Read the model definition and answer for the solid it produces. Units are mm, in the model's axes. Face numbers are marked on the shaded views. A direction names the side the tool comes from. Coordinates: 2 decimals unless noted, no trailing zeros. Write each loop counter-clockwise with the first axis right and the second up, starting at its lowest first coordinate (ties: lowest second). Pieces come first, ordered by that corner, then holes. Notation, with made-up numbers: (81, 70.5) - (127, 70.5) arc R9 ccw to (127, 78.5) - close; hole circle Ø11 at (44.25, -31.75). An arc over 180 degrees is marked (long way). Return JSON: item names as keys, results as strings.
```python
from build123d import *

# Parameters (mm, degrees)
F0_R            = 7.874
F0_R_2          = 6.985
F0_R_3          = 1.397
F1_DEPTH        = 1.27
F2_DEPTH        = 28.575
F4_DEPTH        = 25.4
F4_COPIES_COUNT = 40
F5_SIZE         = 0.254


# Not quite as in the source:
# - a pattern or mirror of a feature is missing from the dataset's text; its kind, count and spacing are read off the source's solid


with BuildPart() as f1:
    # F0 (on Front) → F1 (new body, symmetric)
    with BuildSketch(Plane.XZ):
        Circle(F0_R)
        Circle(F0_R_2, mode=Mode.SUBTRACT)
        Circle(F0_R_2)
        Circle(F0_R_3, mode=Mode.SUBTRACT)
    extrude(amount=F1_DEPTH, both=True)

    # F0 (on Front) → F2 (join, symmetric)
    with BuildSketch(Plane.XZ):
        Circle(F0_R_3)
    extrude(amount=F2_DEPTH, both=True)

    # F3 (on face) → F4 (cut)
    with BuildSketch(Plane.XZ.offset(1.27)):
        with BuildLine():
            ThreePointArc((0.444322899, 7.861453629), (0, 7.874), (-0.444322899, 7.861453629))
            ThreePointArc((-0.444322899, 7.861453629), (0, 7.4295), (0.444322899, 7.861453629))
        make_face()
    f4 = extrude(amount=-F4_DEPTH, mode=Mode.SUBTRACT)

    # F4_copies: F4 ×40 about axis
    f4_copies_axis = Axis((0, 0, 0), (0, 1, 0))
    for i in range(1, F4_COPIES_COUNT):
        add(f4.rotate(f4_copies_axis, i * 360 / F4_COPIES_COUNT), mode=Mode.SUBTRACT)

    # F5
    f5_edges = [f1.edges().sort_by_distance(p)[0] for p in [
        (-1.397, -28.575, 0),
        (-1.397, 28.575, 0),
    ]]
    chamfer(f5_edges, length=F5_SIZE)


solid = f1.part
```
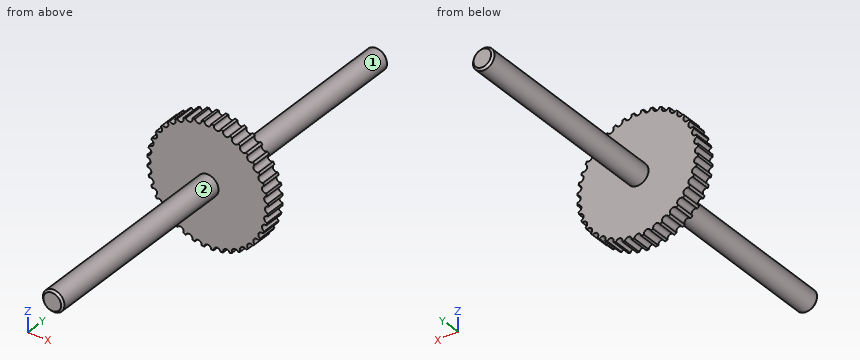
(1) Which of the six approach directions +Z, -Z, +X, -X, +Y, -Y give full straight-line access (tool end or side, diameter ignored) to the marked faces 1 and 2?
Answer:
{"face 1": "+Y", "face 2": "-Y"}
(2) Flat-ended cylindrical pins translate along their axes: P1, Ø3, axis at x = -1, z = 4.5, coming from the +Y side; P2, Ø1.5, axis at x = 5, z = -2, coming from the -Y side; P3, Ø1, axis at x = 0.5, y = -9, coming from the +Z side. Find the tip coordinate at first contact, or state that the pin passes through.
Answer:
{"P1": "y = 1.27", "P2": "y = -1.27", "P3": "z = 1.4"}
(3) Straight lines are drawn through the part: line 1 (Y direction, x = 0.25, z = 6); line 2 (X direction, y = -0.5, z = -6.5); line 3 (Z direction, x = -0.75, y = 19.5). For each, find the intervals that lie inside material, in ascending order. Write a range as from..to.
Answer:
{"line 1": "-1.27..1.27", "line 2": "-4.2..4.2", "line 3": "-1.18..1.18"}
(4) A cutting plane is placed at A-A (y = 14). Determine the outline of the cut face in (x, z), and give its area (3 significant figures).
Answer:
{"outline": "circle Ø2.79 at (0, 0)", "area": "6.13 mm²"}
